Check sheet for the modelled part. Datum: model origin and axes. Units: mm. Face numbers are marked on the shaded views. A direction names the side the tool comes from. Give positions to 0.01 mm unless a question says otherwise; leave off trailing zeros. Loops run counter-clockwise (first coordinate to the right, second up) from the corner with the lowest first, then second, coordinate; pieces in that order, holes last. Notation, with made-up numbers: (56.5, 10.5) -> (62.5, 10.5) arc R21 cw to (62.5, 37.5) -> close; hole circle Ø10 at (-6.75, 72). An arc over 180 degrees is marked (long way). Answer as CSV lines item,"result". Start each with the question number.
(1) Section check D-D on y = 6. Enter the section's corners in (x, z).
(2) Material ranges on line 1 (Z direction, x = 46, y = 31); line 2 (X direction, y = 30.15, z = -15); line 3 (X direction, y = 30.7, z = -15), recorded low to high. Write a range as from..to.
(3) Section check C-C on z = -15. Enter the section's corners in (x, y), plus the area to 3 significant figures.
(4) Section check B-B on y = 22. Enter the section's corners in (x, z), plus the area to 3 significant figures.
(5) Release check for a two-part mould opening along X. For the marked faces 1, 2 and 3 record: pulls with the +X half, pulls with the -X half, needs draft (parallel to the pull), parting line crosses it, or undercut.
(6) Access from +Z, -Z, +X, -X, +Y, -Y to the whole of each face (thin tool, end or side, straight path). Record for the marked faces 4, 5 and 6.
(7) Gauge pin test, flat ends, axial feed: pin 1 Ø3.5 at (x, z) = (0, -13.5) entering from +Y; pin 2 Ø6 at (x, z) = (-46, -15) entering from -Y; pin 3 Ø4 at (x, z) = (-11, -21) entering from +Y; pin 4 Ø8 at (y, z) = (19, -22) entering from -X. Record the tip position at first contact, or that the pin passes through.
(8) Section check A-A on x = -46. Enter the section's corners in (y, z), plus the area to 3 significant figures.
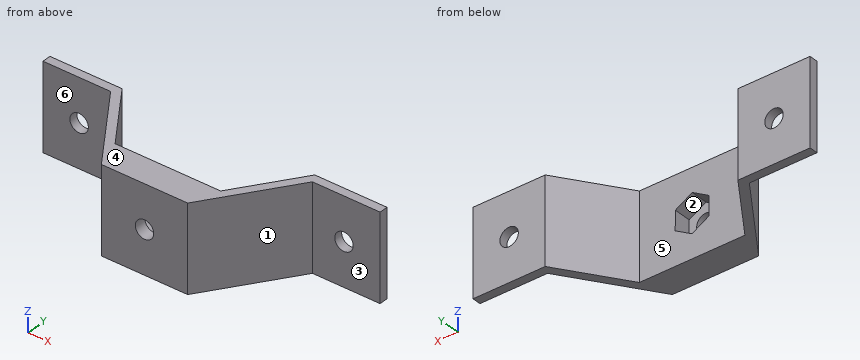
from build123d import *

# Parameters (mm, degrees)
BOSS_EXTRUDE1_DEPTH = 30
SKETCH2_R           = 3.2
CUT_EXTRUDE1_DEPTH  = 3
CUT_EXTRUDE2_REACH  = 12.16
SKETCH5_R           = 3.2
CUT_EXTRUDE3_DEPTH  = 6


with BuildPart() as part:
    # Sketch1 → Boss-Extrude1 (new body)
    with BuildSketch(Plane.XY):
        Polygon((0, 0), (14.990525772, 0), (35.038513576, 29.16), (58.53955614, 29.16), (58.53955614, 32.16), (33.46044386, 32.16), (18.335075832, 10.16), (0, 10.16), align=None)
    boss_extrude1 = extrude(amount=-BOSS_EXTRUDE1_DEPTH)

    # Mirror1: Boss-Extrude1 across plane
    add(boss_extrude1.mirror(Plane(origin=(0, 10.16, -30), x_dir=(0, 0, 1), z_dir=(-1, 0, 0))))

    # Sketch2 → Cut-Extrude1 (cut)
    with BuildSketch(Plane(origin=(0, 32.16, 0), x_dir=(1, 0, 0), z_dir=(0, 1, 0))):
        with Locations((-46, 15)):
            Circle(SKETCH2_R)
    cut_extrude1 = extrude(amount=-CUT_EXTRUDE1_DEPTH, mode=Mode.SUBTRACT)

    # Mirror2: Cut-Extrude1 across plane
    add(cut_extrude1.mirror(Plane(origin=(0, 0, 0), x_dir=(0, 0, 1), z_dir=(1, 0, 0))), mode=Mode.SUBTRACT)

    # Sketch5 → Cut-Extrude2 (cut, up to next)
    with BuildSketch(Plane(origin=(0, 10.16, 0), x_dir=(1, 0, 0), z_dir=(0, 1, 0)), mode=Mode.PRIVATE) as cut_extrude2_sk1:
        with Locations((0.006129123, 15)):
            Circle(SKETCH5_R)
    cut_extrude2_tool1 = extrude(cut_extrude2_sk1.sketch, amount=-CUT_EXTRUDE2_REACH, mode=Mode.PRIVATE) & part.part
    add(cut_extrude2_tool1.solids().sort_by_distance((0.006129, 10.16, -15))[0], mode=Mode.SUBTRACT)

    # Sketch6 → Cut-Extrude3 (cut)
    with BuildSketch(Plane(origin=(0, 10.16, 0), x_dir=(1, 0, 0), z_dir=(0, 1, 0))):
        Polygon((-5.809462538, 18.418212831), (-5.861925855, 11.672656299), (-0.046334193, 8.254443467), (5.821720785, 11.581787169), (5.874184102, 18.327343701), (0.05859244, 21.745556533), align=None)
    extrude(amount=-CUT_EXTRUDE3_DEPTH, mode=Mode.SUBTRACT)


solid = part.part
Working result:
1,outline,"(-19.12, -30) -> (19.12, -30) -> (19.12, 0) -> (-19.12, 0) -> close; hole (-5.86, -11.67) -> (-5.81, -18.42) -> (0.06, -21.75) -> (5.87, -18.33) -> (5.82, -11.58) -> (-0.05, -8.25) -> close"
2,line 1,"z = -30..-18.2, -11.8..0"
2,line 2,"x = -58.54..-49.2, -42.8..-32.08, 32.08..42.8, 49.2..58.54"
2,line 3,"x = -58.54..-49.2, -42.8..-32.46, 32.46..42.8, 49.2..58.54"
3,outline,"(-58.54, 29.16) -> (-49.2, 29.16) -> (-49.2, 32.16) -> (-58.54, 32.16) -> close; (-42.8, 29.16) -> (-35.04, 29.16) -> (-14.99, 0) -> (-3.19, 0) -> (-3.19, 4.16) -> (-5.84, 4.16) -> (-5.84, 10.16) -> (-18.34, 10.16) -> (-33.46, 32.16) -> (-42.8, 32.16) -> close; (3.21, 0) -> (14.99, 0) -> (35.04, 29.16) -> (42.8, 29.16) -> (42.8, 32.16) -> (33.46, 32.16) -> (18.34, 10.16) -> (5.85, 10.16) -> (5.85, 4.16) -> (3.21, 4.16) -> close; (49.2, 29.16) -> (58.54, 29.16) -> (58.54, 32.16) -> (49.2, 32.16) -> close"
3,area,"535 mm^2"
4,outline,"(-30.12, -30) -> (-26.48, -30) -> (-26.48, 0) -> (-30.12, 0) -> close; (26.48, -30) -> (30.12, -30) -> (30.12, 0) -> (26.48, 0) -> close"
4,area,"218 mm^2"
5,face 1,"pulls with the +X half"
5,face 2,"undercut"
5,face 3,"needs draft"
6,face 4,"+Z, +X, -X, +Y, -Y"
6,face 5,"+Z, -Z, +Y"
6,face 6,"+Z, -Z, -X, -Y"
7,pin 1,"stops at y = 4.16"
7,pin 2,"passes through"
7,pin 3,"stops at y = 10.16"
7,pin 4,"stops at x = -30.8"
8,outline,"(29.16, -30) -> (32.16, -30) -> (32.16, -18.2) -> (29.16, -18.2) -> close; (29.16, -11.8) -> (32.16, -11.8) -> (32.16, 0) -> (29.16, 0) -> close"
8,area,"70.8 mm^2"
